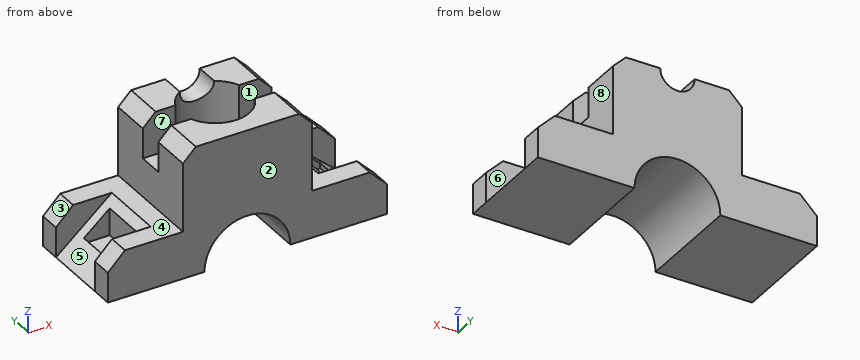
from build123d import *

# Parameters (mm, degrees)
F1_DEPTH  = 50
F2_SIZE   = 8
F3_SIZE   = 6
F4_W      = 6
F4_H      = 12
F5_DEPTH  = 20
F6_R      = 16
F7_DEPTH  = 30
F8_R      = 8
F9_DEPTH  = 25.4
F10_W     = 110.0508913994
F10_H     = 30
F11_DEPTH = 22.001
F12_W     = 112.4475047588
F12_H     = 30
F13_DEPTH = 22.001
F15_DEPTH = 30
F17_DEPTH = 30
F18_W     = 12
F18_H     = 20
F19_DEPTH = 16
F20_W     = 12
F20_H     = 20
F21_DEPTH = 16
F22_R     = 20
F23_DEPTH = 50.0010001


with BuildPart() as f1:
    # F0 (on Front) → F1 (new body)
    with BuildSketch(Plane.XZ):
        Polygon((-65, -8), (-65, -30), (65, -30), (65, -8), (30, -8), (30, 30), (-30, 30), (-30, -8), align=None)
    extrude(amount=F1_DEPTH)

    # F2
    f2_edges = [f1.edges().sort_by_distance(p)[0] for p in [
        (-65, -25, -8),
        (65, -25, -8),
    ]]
    chamfer(f2_edges, length=F2_SIZE)

    # F3
    f3_edges = [f1.edges().sort_by_distance(p)[0] for p in [
        (-30, -25, 30),
        (30, -25, 30),
    ]]
    chamfer(f3_edges, length=F3_SIZE)

    # F4 (on face) → F5 (cut)
    with BuildSketch(Plane.XY.offset(30)):
        with Locations((-27, -25)):
            Rectangle(F4_W, F4_H)
        with Locations((27, -25)):
            Rectangle(F4_W, F4_H)
        with BuildLine():
            Line((-24, -19), (-24, -31))
            Line((-24, -31), (-14.8323969742, -31))
            ThreePointArc((-14.8323969742, -31), (-16, -25), (-14.8323969742, -19))
            Line((-14.8323969742, -19), (-24, -19))
        make_face()
        with BuildLine():
            ThreePointArc((16, -25), (15.70538684, -28.0562761993), (14.8323969742, -31))
            Line((14.8323969742, -31), (24, -31))
            Line((24, -31), (24, -19))
            Line((24, -19), (14.8323969742, -19))
            ThreePointArc((14.8323969742, -19), (15.70538684, -21.9437238007), (16, -25))
        make_face()
    extrude(amount=-F5_DEPTH, mode=Mode.SUBTRACT)

    # F6 (on face) → F7 (cut)
    with BuildSketch(Plane.XY.offset(30)):
        with Locations((0, -25)):
            Circle(F6_R)
    extrude(amount=-F7_DEPTH, mode=Mode.SUBTRACT)

    # F8 (on face) → F9 (cut)
    with BuildSketch(Plane(origin=(0, 0, 0), x_dir=(-1, 0, 0), z_dir=(0, 1, 0))):
        with Locations((0, 30)):
            Circle(F8_R)
    extrude(amount=-F9_DEPTH, mode=Mode.SUBTRACT)

    # F10 (on face) → F11 (cut, through all)
    with BuildSketch(Plane.XY.offset(-8)):
        with Locations((-94.0254456997, -25)):
            Rectangle(F10_W, F10_H)
    extrude(amount=-F11_DEPTH, mode=Mode.SUBTRACT)

    # F12 (on face) → F13 (cut, through all)
    with BuildSketch(Plane.XY.offset(-8)):
        with Locations((95.2237523794, -25)):
            Rectangle(F12_W, F12_H)
    extrude(amount=-F13_DEPTH, mode=Mode.SUBTRACT)

    # F14 (on face) → F15 (join)
    with BuildSketch(Plane.XZ.offset(10)):
        Polygon((39, -30), (65, -30), (39, -8), align=None)
    extrude(amount=F15_DEPTH)

    # F16 (on face) → F17 (join)
    with BuildSketch(Plane.XZ.offset(10)):
        Polygon((-65, -30), (-39, -30), (-39, -8), align=None)
    extrude(amount=F17_DEPTH)

    # F18 (on face) → F19 (cut)
    with BuildSketch(Plane.XY.offset(-8)):
        with Locations((49, -25)):
            Rectangle(F18_W, F18_H)
    extrude(amount=-F19_DEPTH, mode=Mode.SUBTRACT)

    # F20 (on face) → F21 (cut)
    with BuildSketch(Plane.XY.offset(-8)):
        with Locations((-49, -25)):
            Rectangle(F20_W, F20_H)
    extrude(amount=-F21_DEPTH, mode=Mode.SUBTRACT)

    # F22 (on face) → F23 (cut, through all)
    with BuildSketch(Plane.XZ.offset(50)):
        with Locations((0, -30)):
            Circle(F22_R)
    extrude(amount=-F23_DEPTH, mode=Mode.SUBTRACT)


solid = f1.part
Check sheet for the modelled part. Datum: model origin and axes. Units: mm. Face numbers are marked on the shaded views. A direction names the side the tool comes from. Give positions to 0.01 mm unless a question says otherwise; leave off trailing zeros. Write each loop counter-clockwise with the first axis right and the second up, starting at its lowest first coordinate (ties: lowest second). Pieces come first, ordered by that corner, then holes. Notation, with made-up numbers: (-2, 12.25) -> (29, 12.25) arc R27 cw to (29, 32.25) -> close; hole circle Ø5 at (19, 50.25). An arc over 180 degrees is marked (long way). Use one line per item in the form item = value. Start each with the question number.
1. Access from +Z, -Z, +X, -X, +Y, -Y to the whole of each face (thin tool, end or side, straight path). Record for the marked faces 4, 5, 6, 7 and 8.
2. Section check D-D (z = 2). Record the cut outline in (x, y).
3. Section check B-B (y = -25). Record the cut outline in (x, z), and give its area (3 significant figures).
4. Section check C-C (x = 0). Record the cut outline in (y, z), and give its area (3 significant figures).
5. Thickness scan on line 1 along X through (y, z) = (-25, 8); line 2 along Y through (x, z) = (0, 10.5); line 3 along Y through (x, z) = (59, -22.5). Record the ranges inside material, lowest first. Write a range as from..to.
6. Go/stop test with flat-tipped pins: P1, Ø3.5, axis at x = -51.5, y = -29, coming from the +Z side; P2, Ø10, axis at y = -24.5, z = -15, coming from the +X side; P3, Ø8, axis at y = -9, z = 20, coming from the +X side. Record where each tip stops, or that it passes through.
7. Section check A-A (z = 15). Record the cut outline in (x, y), and give its area (3 significant figures).
8. Mould release check, pull along Y, two halves, no side actions. Record for the marked faces 1, 2 and 3: pulls with the +Y half, pulls with the -Y half, needs draft (parallel to the pull), parting line crosses it, or undercut.
Conclusion:
q1.face_4 = +Z, -X, +Y, -Y
q1.face_5 = +Z, -X
q1.face_6 = +Z, +X
q1.face_7 = +Z, +X, -X
q1.face_8 = +Z, +X, +Y, -Y
q2.outline = (-30, -50) -> (30, -50) -> (30, 0) -> (-30, 0) -> close; hole circle Ø32 at (0, -25)
q3.outline = (-65, -30) -> (-20, -30) arc R20 cw to (20, -30) -> (65, -30) -> (55, -21.54) -> (55, -24) -> (43, -24) -> (43, -11.38) -> (39, -8) -> (30, -8) -> (30, 10) -> (16, 10) -> (16, 0) -> (-16, 0) -> (-16, 10) -> (-30, 10) -> (-30, -8) -> (-39, -8) -> (-43, -11.38) -> (-43, -24) -> (-55, -24) -> (-55, -21.54) -> close
q3.area = 2,240 mm²
q4.outline = (-50, -10) -> (0, -10) -> (0, 22) -> (-9, 22) -> (-9, 0) -> (-41, 0) -> (-41, 30) -> (-50, 30) -> close
q4.area = 968 mm²
q5.line_1 = -30..-16, 16..30
q5.line_2 = -50..-41, -9..0
q5.line_3 = -50..-40, -10..0
q6.P1 = -24
q6.P2 = 43
q6.P3 = 30
q7.outline = (-30, -50) -> (30, -50) -> (30, -31) -> (14.83, -31) arc R16 cw to (-14.83, -31) -> (-30, -31) -> close; (-30, -19) -> (-14.83, -19) arc R16 cw to (14.83, -19) -> (30, -19) -> (30, 0) -> (-30, 0) -> close
q7.area = 1,850 mm²
q8.face_1 = undercut
q8.face_2 = pulls with the -Y half
q8.face_3 = needs draft
